from build123d import *
from build123d.topology import SkipClean

# Parameters (mm, degrees)
SKETCH1_W           = 123
SKETCH1_H           = 110
BOSS_EXTRUDE1_DEPTH = 20
CUT_EXTRUDE3_DEPTH  = 150
FILLET2_R           = 5
FILLET5_R           = 15
FILLET6_SIZE        = 2
FILLET6_SIZE_2      = 3
FILLET7_SIZE        = 2
FILLET7_SIZE_2      = 3
FILLET8_R           = 5
BOSS_EXTRUDE3_START = -18
SKETCH6_W           = 113
SKETCH6_H           = 14.5
BOSS_EXTRUDE3_DEPTH = 64
CUT_EXTRUDE4_DEPTH  = 64
FILLET10_R          = 4
BOSS_EXTRUDE4_DEPTH = 10


# Some blends are built 0.0001 mm under size
with BuildPart() as part:
    # Sketch1 → Boss-Extrude1 (new body)
    with BuildSketch(Plane(origin=(0, 0, 0), x_dir=(1, 0, 0), z_dir=(0, 1, 0))):
        with Locations((53.726554268, 129.299262381)):
            Rectangle(SKETCH1_W, SKETCH1_H)
    extrude(amount=BOSS_EXTRUDE1_DEPTH)

    # Sketch5 → Cut-Extrude3 (cut)
    with BuildSketch(Plane.XY.offset(-74.299262381)):
        Polygon((5.893432633, 20), (101.559675903, 20), (108.776554268, 7.5), (-1.323445732, 7.5), align=None)
    extrude(amount=-CUT_EXTRUDE3_DEPTH, mode=Mode.SUBTRACT)

    # Fillet2
    fillet2_edges = [part.edges().sort_by_distance(p)[0] for p in [
        (108.776554268, 7.5, -129.299262381),
        (-1.323445732, 7.5, -129.299262381),
    ]]
    fillet(fillet2_edges, radius=FILLET2_R)

    # Fillet5
    fillet5_edges = [part.edges().sort_by_distance(p)[0] for p in [
        (115.226554268, 0, -129.299262381),
        (-7.773445732, 0, -129.299262381),
    ]]
    fillet(fillet5_edges, radius=FILLET5_R)

    # Fillet6
    # an asymmetric fillet: 3, 2 mm, written as the material it takes off along each edge
    with BuildSketch(Plane(origin=(3.006681287, 15, -74.299262381), x_dir=(-0.8660254037844386, 0.5000000000000001, 0), z_dir=(0.5000000000000001, 0.8660254037844387, 0)), Plane(origin=(97.809675903, 26.495190529, -74.299262381), x_dir=(0.8660254037844344, 0.5000000000000074, 0), z_dir=(0.5000000000000074, -0.8660254037844345, 0))) as fillet6_piece_1:
        with BuildLine():
            Bezier((FILLET6_SIZE, 0), (0, 0), (0, -FILLET6_SIZE_2), weights=[1, 0.707106781, 1])
            Line((0, -FILLET6_SIZE_2), (0, 0))
            Line((0, 0), (FILLET6_SIZE, 0))
        make_face()
    extrude(amount=13.273502692, mode=Mode.SUBTRACT)
    with BuildSketch(Plane(origin=(7.336808305, 12.5, -74.299262381), x_dir=(0, -1, 0), z_dir=(1, 0, 0))) as fillet6_piece_2:
        with BuildLine():
            Bezier((5 + FILLET6_SIZE, 0), (5, 0), (5, FILLET6_SIZE_2), weights=[1, 0.707106781, 1])
            Line((5, FILLET6_SIZE_2), (5, 0))
            Line((5, 0), (5 + FILLET6_SIZE, 0))
        make_face()
    revolve(axis=Axis((7.336808305, 12.5, -74.299262381), (0, 0, -1)), revolution_arc=120, mode=Mode.SUBTRACT)
    with BuildSketch(Plane(origin=(100.11630023, 12.5, -74.299262381), x_dir=(0.8660254037844343, 0.5000000000000077, 0), z_dir=(-0.5000000000000077, 0.8660254037844343, 0))) as fillet6_piece_3:
        with BuildLine():
            Bezier((5 + FILLET6_SIZE, 0), (5, 0), (5, FILLET6_SIZE_2), weights=[1, 0.707106781, 1])
            Line((5, FILLET6_SIZE_2), (5, 0))
            Line((5, 0), (5 + FILLET6_SIZE, 0))
        make_face()
    revolve(axis=Axis((100.11630023, 12.5, -74.299262381), (0, 0, -1)), revolution_arc=120, mode=Mode.SUBTRACT)
    with BuildSketch(Plane(origin=(100.11630023, 7.5, -74.299262381), x_dir=(0, -1, 0), z_dir=(-1, 0, 0))) as fillet6_piece_4:
        with BuildLine():
            Bezier((FILLET6_SIZE, 0), (0, 0), (0, -FILLET6_SIZE_2), weights=[1, 0.707106781, 1])
            Line((0, -FILLET6_SIZE_2), (0, 0))
            Line((0, 0), (FILLET6_SIZE, 0))
        make_face()
    extrude(amount=92.779491924, mode=Mode.SUBTRACT)

    # Fillet7
    # an asymmetric fillet: 3, 2 mm, written as the material it takes off along each edge
    with BuildSketch(Plane(origin=(3.006681287, 15, -184.299262381), x_dir=(-0.8660254037844386, 0.5000000000000001, 0), z_dir=(0.5000000000000001, 0.8660254037844387, 0)), Plane(origin=(97.809675903, 26.495190528, -184.299262381), x_dir=(0.8660254037844344, 0.5000000000000074, 0), z_dir=(0.5000000000000074, -0.8660254037844345, 0))) as fillet7_piece_1:
        with BuildLine():
            Bezier((FILLET7_SIZE, 0), (0, 0), (0, FILLET7_SIZE_2), weights=[1, 0.707106781, 1])
            Line((0, FILLET7_SIZE_2), (0, 0))
            Line((0, 0), (FILLET7_SIZE, 0))
        make_face()
    extrude(amount=13.273502692, mode=Mode.SUBTRACT)
    with BuildSketch(Plane(origin=(7.336808305, 12.5, -184.299262381), x_dir=(0, -1, 0), z_dir=(1, 0, 0))) as fillet7_piece_2:
        with BuildLine():
            Bezier((5 + FILLET7_SIZE, 0), (5, 0), (5, -FILLET7_SIZE_2), weights=[1, 0.707106781, 1])
            Line((5, -FILLET7_SIZE_2), (5, 0))
            Line((5, 0), (5 + FILLET7_SIZE, 0))
        make_face()
    revolve(axis=Axis((7.336808305, 12.5, -184.299262381), (0, 0, -1)), revolution_arc=120, mode=Mode.SUBTRACT)
    with BuildSketch(Plane(origin=(100.11630023, 12.5, -184.299262381), x_dir=(0.8660254037844343, 0.5000000000000077, 0), z_dir=(-0.5000000000000077, 0.8660254037844343, 0))) as fillet7_piece_3:
        with BuildLine():
            Bezier((5 + FILLET7_SIZE, 0), (5, 0), (5, -FILLET7_SIZE_2), weights=[1, 0.707106781, 1])
            Line((5, -FILLET7_SIZE_2), (5, 0))
            Line((5, 0), (5 + FILLET7_SIZE, 0))
        make_face()
    revolve(axis=Axis((100.11630023, 12.5, -184.299262381), (0, 0, -1)), revolution_arc=120, mode=Mode.SUBTRACT)
    with BuildSketch(Plane(origin=(100.11630023, 7.5, -184.299262381), x_dir=(0, -1, 0), z_dir=(-1, 0, 0))) as fillet7_piece_4:
        with BuildLine():
            Bezier((FILLET7_SIZE, 0), (0, 0), (0, FILLET7_SIZE_2), weights=[1, 0.707106781, 1])
            Line((0, FILLET7_SIZE_2), (0, 0))
            Line((0, 0), (FILLET7_SIZE, 0))
        make_face()
    extrude(amount=92.779491924, mode=Mode.SUBTRACT)

    # Fillet8
    fillet8_edges = [part.edges().sort_by_distance(p)[0] for p in [
        (-7.773445732, 20, -129.299262381),
        (115.226554268, 20, -129.299262381),
    ]]
    fillet(fillet8_edges, radius=FILLET8_R - 0.0001)  # a hair under: the kernel refuses the full size

    # Sketch6 → Boss-Extrude3 (add)
    with BuildSketch(Plane(origin=(0, 0, -184.299262381), x_dir=(-1, 0, 0), z_dir=(0, 0, -1)).offset(BOSS_EXTRUDE3_START)):
        with Locations((-53.726554268, 12.75)):
            Rectangle(SKETCH6_W, SKETCH6_H)
    extrude(amount=-BOSS_EXTRUDE3_DEPTH)

    # Sketch8 → Cut-Extrude4 (cut)
    with BuildSketch(Plane.XY.offset(-102.299262381)):
        Polygon((1.226554268, 9), (106.226554268, 9), (99.875701307, 20), (7.577407229, 20), align=None)
    extrude(amount=-CUT_EXTRUDE4_DEPTH, mode=Mode.SUBTRACT)

    # Fillet10
    # the kernel refuses this fillet: 4 mm, written as the material it adds along each edge
    with BuildSketch(Plane(origin=(1.226554268, 9, -102.299262381), x_dir=(0.5000000000000043, 0.8660254037844362, 0), z_dir=(0, 0, -1))) as fillet10_piece_1:
        with BuildLine():
            CenterArc((FILLET10_R * 1.73205080757, FILLET10_R), FILLET10_R, 150, 120)
            Line((FILLET10_R * 0.866025403784, FILLET10_R * 1.5), (0, 0))
            Line((0, 0), (FILLET10_R * 1.73205080757, 0))
        make_face()
    extrude(amount=64)
    with BuildSketch(Plane(origin=(106.226554268, 9, -102.299262381), x_dir=(-0.5000000000000053, 0.8660254037844355, 0), z_dir=(0, 0, -1))) as fillet10_piece_2:
        with BuildLine():
            CenterArc((FILLET10_R * 1.73205080757, -FILLET10_R), FILLET10_R, 90, 120)
            Line((FILLET10_R * 0.866025403784, -FILLET10_R * 1.5), (0, 0))
            Line((0, 0), (FILLET10_R * 1.73205080757, 0))
        make_face()
    extrude(amount=64)

    # Sketch9 → Boss-Extrude4 (add)
    with SkipClean():  # the faces are left unmerged after this step: merging them gives an invalid solid
        with BuildSketch(Plane.XY.offset(-102.299262381)):
            with BuildLine():
                Line((8.154757498, 9), (99.298351037, 9))
                ThreePointArc((99.298351037, 9), (102.762452653, 11), (102.762452653, 15))
                Line((102.762452653, 15), (99.875701307, 20))
                Line((99.875701307, 20), (101.559675903, 20))
                Line((101.559675903, 20), (104.446427249, 15))
                ThreePointArc((104.446427249, 15), (104.446427249, 10), (100.11630023, 7.5))
                Line((100.11630023, 7.5), (7.336808305, 7.5))
                ThreePointArc((7.336808305, 7.5), (3.014687704, 9.986183479), (2.990801035, 14.972290599))
                ThreePointArc((2.990801035, 14.972290599), (2.998719037, 14.986157979), (3.006681287, 15))
                Line((3.006681287, 15), (5.893432633, 20))
                Line((5.893432633, 20), (7.577407229, 20))
                Line((7.577407229, 20), (4.690655883, 15))
                ThreePointArc((4.690655883, 15), (4.690655883, 11), (8.154757498, 9))
            make_face()
        extrude(amount=BOSS_EXTRUDE4_DEPTH)


solid = part.part
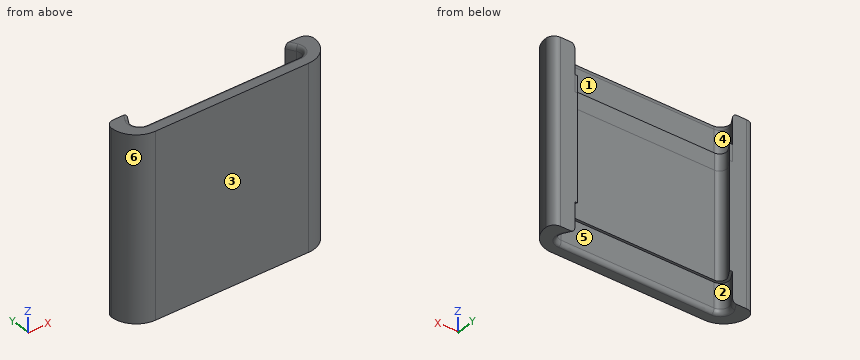
CAD build for the part. Positions are in the model's coordinates, mm. Face numbers are marked on the shaded views. A direction names the side the tool comes from. Round coordinates to 2 decimals unless told otherwise and drop trailing zeros. Order: outer loops, then holes, each group sorted by start corner. A loop starts at its lowest first (then second) coordinate and runs counter-clockwise, first axis right, second up. Notation, with made-up numbers: (53, 31.5) -> (73, 31.5) arc R6 cw to (73, 41.5) -> close; hole circle Ø5 at (-5, -28.5). An arc over 180 degrees is marked (long way). Write each question's results on one line, items separated by ' | '.
1. Cut at C-C (y = 3.25). Give the cut face in (x, z).
Findings below:
outline: (-2.1, -184.3) -> (109.55, -184.3) -> (109.55, -74.3) -> (-2.1, -74.3) -> close
2. Wall check: line 1 along Z through (x, y) = (103, 9.25); line 2 along Y through (x, z) = (24, -120); line 3 along X through (y, z) = (18.75, -156). Give the ranges that are in metal, low to high. Write a range as [from, to].
Findings below:
line 1: z = [-166.3, -92.3] | line 2: y = [0, 9] | line 3: x = [-6.08, 6.86], [100.6, 113.53]
3. Flat gauge pins, fed straight in: P1, Ø2, axis at x = 102.5, y = 12, coming from the +Z side; P2, Ø7.5, axis at x = 49, z = -176, coming from the +Y side; P3, Ø8, axis at y = 8.5, z = -139.5, coming from the +X side. Where does each tip first touch, or does it go through?
Findings below:
P1: stops at z = -92.3 | P2: stops at y = 7.5 | P3: stops at x = 115.02
4. Pull direction Y, two halves, no side cores. Call the marked faces 1, 2 and 3: pulls with the +Y half, pulls with the -Y half, needs draft (parallel to the pull), parting line crosses it, or undercut.
Findings below:
face 1: pulls with the +Y half | face 2: undercut | face 3: pulls with the -Y half
5. 3-axis set-ups, long thin cutter, end or side, ignore diameter. For the marked faces 4, 5 and 6: which of +Z, -Z, +X, -X, +Y, -Y reach the whole face in a straight line?
Findings below:
face 4: +Z | face 5: -Z, +Y | face 6: +Z, -Z, -X, -Y
